Verification items for this drawing (mm, ordinates from the low corner). Coordinates: 2 decimals unless noted, no trailing zeros. Loops run counter-clockwise (first coordinate to the right, second up) from the corner with the lowest first, then second, coordinate; pieces in that order, holes last. Notation, with made-up numbers: (73.5, 23) - (109.5, 23) arc R18 cw to (109.5, 55) - close; hole circle Ø3 at (17, 27). An arc over 180 degrees is marked (long way). Write each question's results on one line, items separated by ' | '. Start each with the question number.
(1) Sectioned sample at A-A (x = 71). Enter the section's corners in (y, z), plus the area to 3 significant figures.
(2) Sectioned sample at D-D (y = 4.75). Enter the section's corners in (x, z), plus the area to 3 significant figures.
(3) Material ranges on probe 1 along Z at (x, y) = (41, 4); probe 2 along X at (y, z) = (1.5, 41); probe 3 along X at (y, z) = (2.25, 25.5), recorded low to high.
(4) Sectioned sample at C-C (x = 41). Enter the section's corners in (y, z).
(5) Sectioned sample at B-B (z = 25.5). Enter the section's corners in (x, y).
(6) Mould release check, pull along X, two halves, no side actions. Record for the marked faces 1 and 2: pulls with the +X half, pulls with the -X half, needs draft (parallel to the pull), parting line crosses it, or undercut.
(7) Go/stop test with flat-tipped pins: pin 1 Ø1.8 at (x, z) = (10, 10) entering from -Y; pin 2 Ø3 at (y, z) = (4.5, 15) entering from +X. Record where each tip stops, or that it passes through.
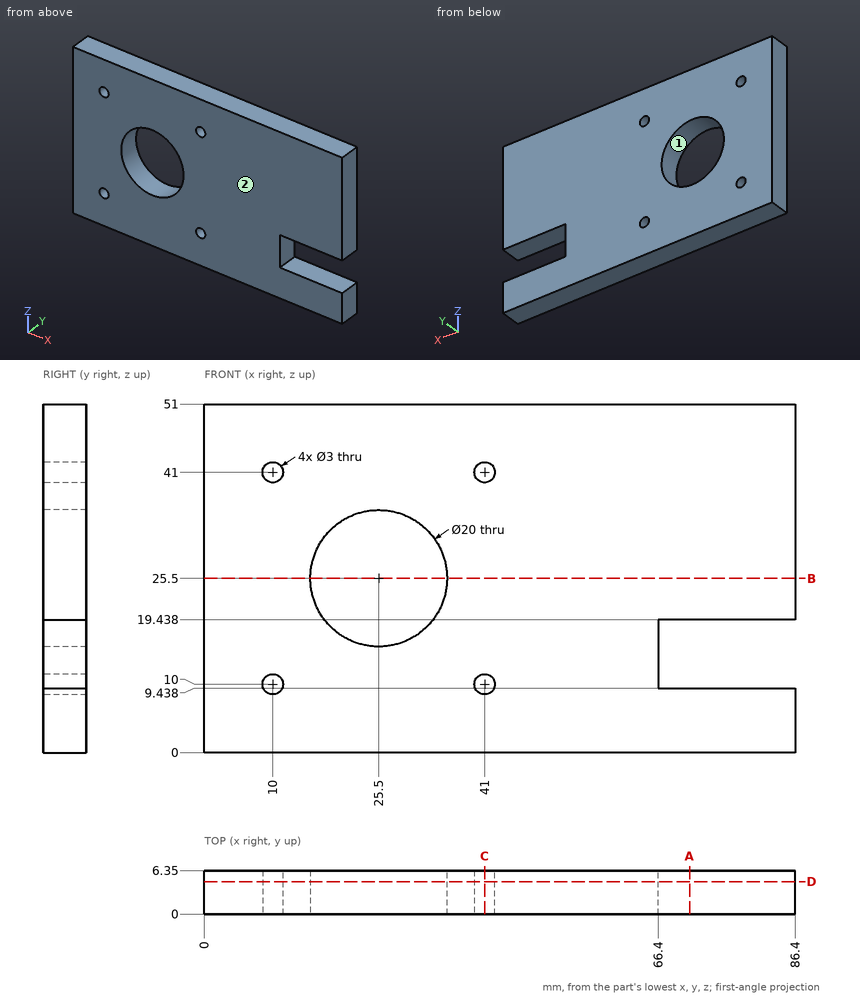
Outcome:
1) outline: (0, 0) - (6.35, 0) - (6.35, 9.44) - (0, 9.44) - close; (0, 19.44) - (6.35, 19.44) - (6.35, 51) - (0, 51) - close | area: 260 mm2
2) outline: (0, 0) - (86.4, 0) - (86.4, 9.44) - (66.4, 9.44) - (66.4, 19.44) - (86.4, 19.44) - (86.4, 51) - (0, 51) - close; hole circle Ø3 at (10, 10); hole circle Ø3 at (10, 41); hole circle Ø20 at (25.5, 25.5); hole circle Ø3 at (41, 10); hole circle Ø3 at (41, 41) | area: 3,860 mm2
3) probe 1: z = 0 to 8.5, 11.5 to 39.5, 42.5 to 51 | probe 2: x = 0 to 8.5, 11.5 to 39.5, 42.5 to 86.4 | probe 3: x = 0 to 15.5, 35.5 to 86.4
4) outline: (0, 0) - (6.35, 0) - (6.35, 8.5) - (0, 8.5) - close; (0, 11.5) - (6.35, 11.5) - (6.35, 39.5) - (0, 39.5) - close; (0, 42.5) - (6.35, 42.5) - (6.35, 51) - (0, 51) - close
5) outline: (0, 0) - (15.5, 0) - (15.5, 6.35) - (0, 6.35) - close; (35.5, 0) - (86.4, 0) - (86.4, 6.35) - (35.5, 6.35) - close
6) face 1: undercut | face 2: needs draft
7) pin 1: passes through | pin 2: stops at x = 66.4
